Check sheet for the drawn part. Datum: minimum x, y, z corner. Units: mm. A direction names the side the tool comes from. Give positions to 0.01 mm unless a question says otherwise; leave off trailing zeros. Order: outer loops, then holes, each group sorted by start corner. A loop starts at its lowest first (then second) coordinate and runs counter-clockwise, first axis right, second up.
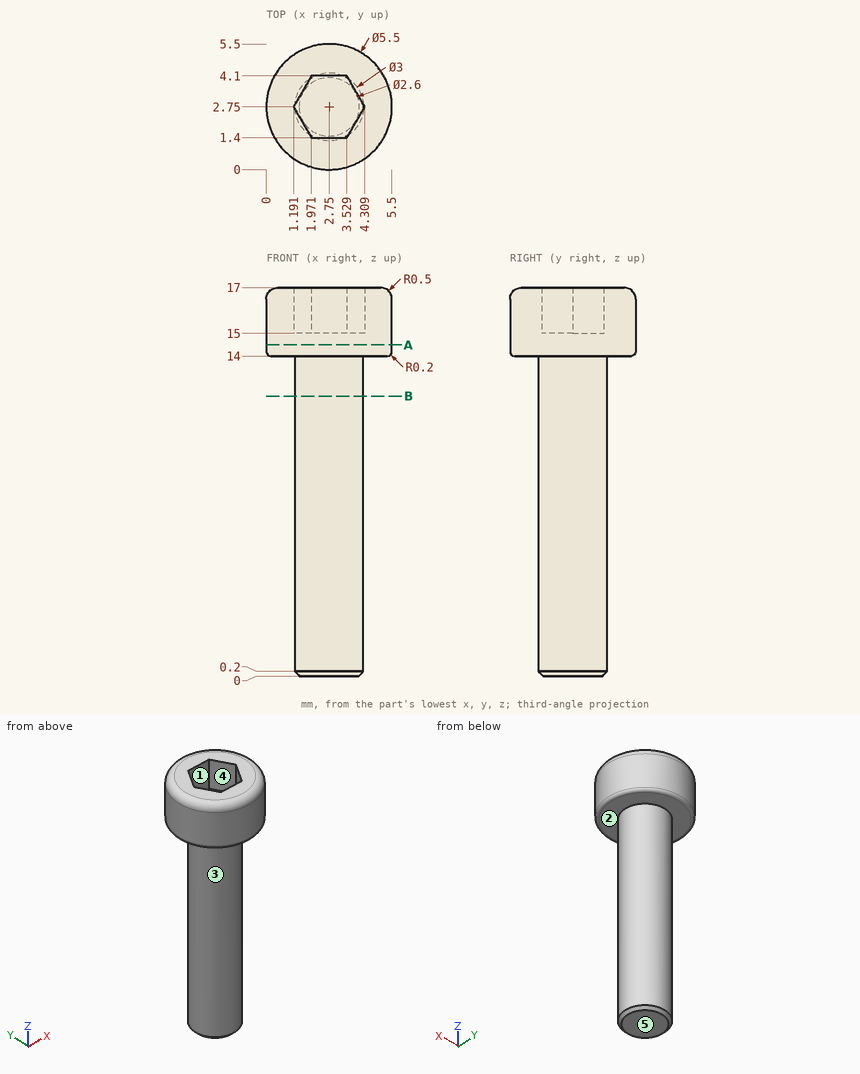
(1) Section check B-B, the plane z = 12.25. Enter the section's corners in (x, y).
Solved:
outline: circle Ø3 at (2.75, 2.75)
(2) Go/stop test with flat-tipped pins: pin 1 (1.4 mm diameter, centred on x = 2, y = 2, fed in from +Z); pin 2 (2 mm diameter, centred on x = 2, z = 4.5, fed in from -Y); pin 3 (1.5 mm diameter, centred on y = 1, z = 5, fed in from +X). Record where each tip stops, or that it passes through.
Solved:
pin 1: stops at z = 17
pin 2: stops at y = 1.25
pin 3: stops at x = 3.87
(3) Scan lines: line 1 (Z direction, x = 4.45, y = 4.15); line 2 (Z direction, x = 3.95, y = 2.6); line 3 (Y direction, x = 3.45, z = 16). Record each from-to range of solid material in increasing order.
Solved:
line 1: z = 14 to 17
line 2: z = 0 to 15
line 3: y = 0.09 to 1.4, 4.1 to 5.41
(4) Section check A-A, the plane z = 14.5. Enter the section's corners in (x, y).
Solved:
outline: circle Ø5.5 at (2.75, 2.75)
(5) Set-up check for the marked faces 4 and 5: record each of +Z, -Z, +X, -X, +Y, -Y from which the full face is reachable in a straight line by a thin tool's end or side.
Solved:
face 4: +Z
face 5: -Z, +X, -X, +Y, -Y
(6) Release check for a two-part mould opening along X. For the marked faces 1, 2 and 3 record: pulls with the +X half, pulls with the -X half, needs draft (parallel to the pull), parting line crosses it, or undercut.
Solved:
face 1: undercut
face 2: needs draft
face 3: parting line crosses it
